For this review, take the finished solid that the model builds, in its own axes (mm). A direction names the side the tool comes from. Round coordinates to 2 decimals unless told otherwise and drop trailing zeros. Write each loop counter-clockwise with the first axis right and the second up, starting at its lowest first coordinate (ties: lowest second). Pieces come first, ordered by that corner, then holes. Notation, with made-up numbers: (1, -32.75) -> (16, -32.75) arc R16 cw to (16, -12.75) -> close; hole circle Ø3 at (62.25, 33). An arc over 180 degrees is marked (long way). Answer as CSV lines item,"result". Start each with the question number.
Item 1: For pin 1 Ø1.8 at (y, z) = (-748.5, -1) entering from +X; pin 2 Ø2 at (x, y) = (7.5, -530) entering from +Z; pin 3 Ø3 at (x, z) = (-26, -1) entering from -Y, all flat-tipped, find the tip position at first contact; note any pin that passes through.
Item 2: Wall thickness on probe 1 along Y at (x, z) = (2, 16.5); probe 2 along Z at (x, y) = (1, -554); probe 3 along X at (y, z) = (-188.5, 0.5): over which ranges is each line inside the solid? List them lowest first. Write a range as from..to.
Item 3: Take a section at B-B on z = -24. Give the boundary of the cut face in (x, y), then the cut area to 3 significant figures.
Item 4: Mouldability with a two-part tool opening along Z and no side actions: class faces 4 (the flat face through (-7.665, -428, -23)), 5 (the cylindrical face through (-32.06, -375.67, 29.4)), 6 (the flat face through (18, -747, -3)) as +Z half, -Z half, draft (parallel to the pull), parting line (faces both ways), or undercut.
Item 5: Machinability: for faces 1 (the flat face through (1.616, -428, 25)), 2 (the flat face through (-22, -85, -17)), 3 (the flat face through (-10, -747, 3)), which of the approach directions +Z, -Z, +X, -X, +Y, -Y give a long, thin tool a straight path to every point of the face, cutting with its end or side? Answer none if there is none.
Item 6: Take a section at C-C on x = -33. Give the boundary of the cut face in (y, z), then the cut area to 3 significant figures.
Item 7: Take a section at A-A on y = -100. Give the boundary of the cut face in (x, z), then the cut area to 3 significant figures.
```python
from build123d import *

# Parameters (mm, degrees)
F0_R     = 43.5
F1_DEPTH = 762
F2_W     = 99
F2_H     = 6
F3_DEPTH = 30
F4_W     = 7.932048
F4_H     = 6
F5_DEPTH = 25
F6_W     = 43.600235
F6_H     = 52.118463
F6_W_2   = 52.118463
F6_H_2   = 43.600235
F7_DEPTH = 677


with BuildPart() as f1:
    # F0 (on Front) → F1 (new body)
    with BuildSketch(Plane.XZ):
        Circle(F0_R)
    extrude(amount=F1_DEPTH)

    # F2 (on face) → F3 (cut)
    with BuildSketch(Plane.XZ.offset(762)):
        Rectangle(F2_W, F2_H)
    extrude(amount=-F3_DEPTH, mode=Mode.SUBTRACT)

    # F4 (on face) → F5 (join)
    with BuildSketch(Plane.XZ.offset(732)):
        Rectangle(F4_W, F4_H)
    extrude(amount=F5_DEPTH)

    # F6 (on face) → F7 (cut)
    with BuildSketch(Plane.XZ.offset(762)):
        with Locations((23.416517, 33.724575)):
            Rectangle(F6_W, F6_H)
        with Locations((-33.724575, -23.416517)):
            Rectangle(F6_W_2, F6_H_2)
    extrude(amount=-F7_DEPTH, mode=Mode.SUBTRACT)


solid = f1.part
```
Output values:
1,pin 1,"stops at x = 3.97"
1,pin 2,"stops at z = 7.67"
1,pin 3,"stops at y = -732"
2,probe 1,"y = -85..0"
2,probe 2,"z = -43.49..43.49"
2,probe 3,"x = -43.5..43.5"
3,outline,"(-36.28, -85) -> (-7.67, -85) -> (-7.67, -762) -> (36.28, -762) -> (36.28, 0) -> (-36.28, 0) -> close"
3,area,"35,900 mm^2"
4,face 4,"draft"
4,face 5,"parting line"
4,face 6,"undercut"
5,face 1,"+Z, +X, -Y"
5,face 2,"-Z, -X, -Y"
5,face 3,"-Y"
6,outline,"(-762, 3) -> (-732, 3) -> (-732, -1.62) -> (-85, -1.62) -> (-85, -28.34) -> (0, -28.34) -> (0, 28.34) -> (-762, 28.34) -> close"
6,area,"25,000 mm^2"
7,outline,"(-43.47, -1.62) -> (-7.67, -1.62) -> (-7.67, -42.82) arc R43.5 ccw to (42.82, 7.67) -> (1.62, 7.67) -> (1.62, 43.47) arc R43.5 ccw to start"
7,area,"3,750 mm^2"
